The figure shows three views and two pictorial views of one solid part (mm, origin at its lowest corner). Answer the questions. A direction names the side the tool comes from. Coordinates: 2 decimals unless noted, no trailing zeros. Order: outer loops, then holes, each group sorted by start corner. A loop starts at its lowest first (then second) coordinate and runs counter-clockwise, first axis right, second up. Notation, with made-up numbers: (-10, -29.75) - (47, -29.75) arc R17 cw to (47, -15.75) - close; hole circle Ø11 at (31.25, 88.5). An arc over 180 degrees is marked (long way). Answer as a JSON object with one key per item and string values. Group by question number.
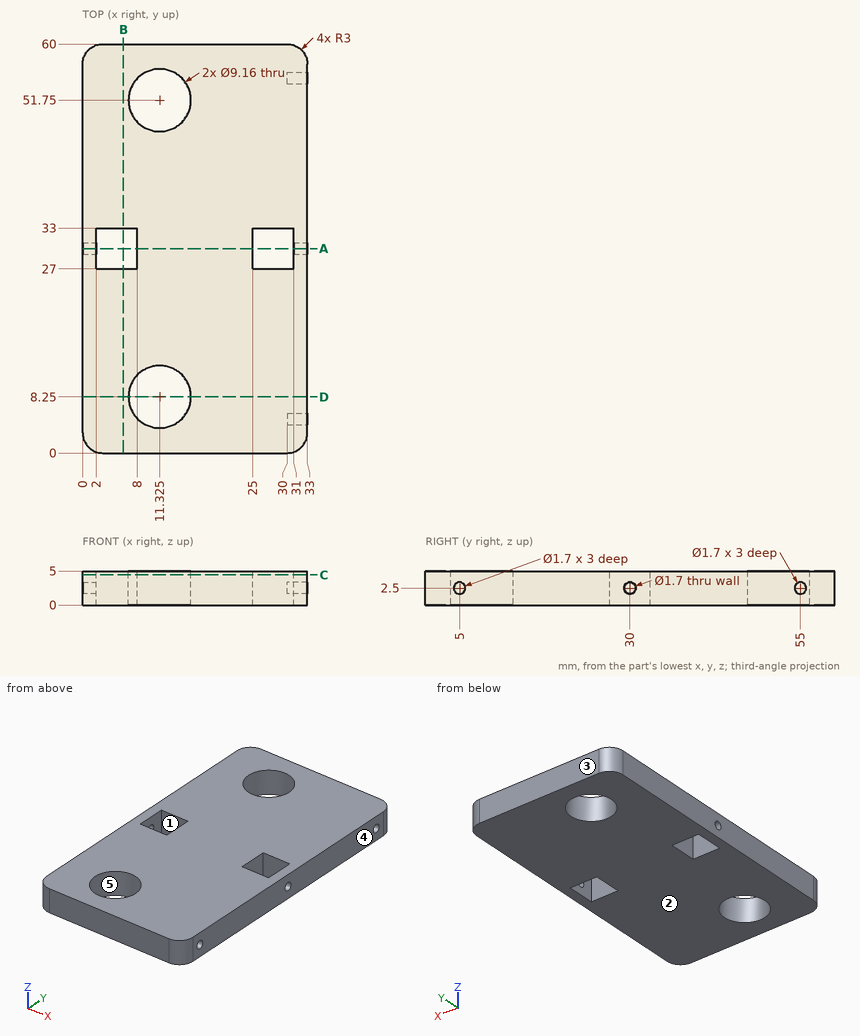
1. A cutting plane is placed at A-A on y = 30. Write down the section's boundary in (x, z).
2. For a pull along Y with two mould halves and no side action, classify the marked faces 3, 4 and 5 as pulls with the +Y half, pulls with the -Y half, needs draft (parallel to the pull), parting line crosses it, or undercut.
3. Given pin 1 (1.4 mm diameter, centred on y = 5, z = 2.5, fed in from +X); pin 2 (8 mm diameter, centred on x = 11.325, y = 51.75, fed in from +Z); pin 3 (1 mm diameter, centred on y = 30, z = 2.5, fed in from -X); pin 4 (1.4 mm diameter, centred on y = 30, z = 2.5, fed in from +X), each flat-ended and moving along its own axis, determine where each tip first touches the part or whether it passes through.
4. A cutting plane is placed at D-D on y = 8.25. Write down the section's boundary in (x, z) (3 decimals), and give its area (3 significant figures).
5. A cutting plane is placed at B-B on x = 6. Write down the section's boundary in (y, z), and give its area (3 significant figures).
6. Straight lines are drawn through the part: L1, parallel to Y at x = 11.5, z = 3.4; L2, parallel to Y at x = 26, z = 2.4; L3, parallel to X at y = 8.5, z = 1.8. For each, find the intervals that lie inside material, in ascending order.
7. For the marked faces 1 and 2, determine the directions among +Z, -Z, +X, -X, +Y, -Y from which every point of the face is accessible in a straight line to the end or side of a thin tool.
8. A cutting plane is placed at C-C on z = 4.45. Write down the section's boundary in (x, y) (3 decimals).
Derived:
{
 "1": {"outline": "(0, 0) - (2, 0) - (2, 1.65) - (0, 1.65) - close; (0, 3.35) - (2, 3.35) - (2, 5) - (0, 5) - close; (8, 0) - (25, 0) - (25, 5) - (8, 5) - close; (31, 0) - (33, 0) - (33, 1.65) - (31, 1.65) - close; (31, 3.35) - (33, 3.35) - (33, 5) - (31, 5) - close"},
 "2": {"face 3": "pulls with the +Y half", "face 4": "needs draft", "face 5": "undercut"},
 "3": {"pin 1": "stops at x = 30", "pin 2": "passes through", "pin 3": "stops at x = 8", "pin 4": "stops at x = 25"},
 "4": {"outline": "(0, 0) - (6.745, 0) - (6.745, 5) - (0, 5) - close; (15.905, 0) - (33, 0) - (33, 5) - (15.905, 5) - close", "area": "119 mm2"},
 "5": {"outline": "(0, 0) - (27, 0) - (27, 5) - (0, 5) - close; (33, 0) - (60, 0) - (60, 5) - (33, 5) - close", "area": "270 mm2"},
 "6": {"L1": "y = 0 to 3.67, 12.83 to 47.17, 56.33 to 60", "L2": "y = 0 to 27, 33 to 60", "L3": "x = 0 to 6.75, 15.9 to 33"},
 "7": {"face 1": "+Z, -Z", "face 2": "-Z, +X, -X, +Y, -Y"},
 "8": {"outline": "(0, 3) arc R3 ccw to (3, 0) - (30, 0) arc R3 ccw to (33, 3) - (33, 57) arc R3 ccw to (30, 60) - (3, 60) arc R3 ccw to (0, 57) - close; hole (2, 27) - (8, 27) - (8, 33) - (2, 33) - close; hole circle Ø9.16 at (11.325, 8.25); hole circle Ø9.16 at (11.325, 51.75); hole (25, 27) - (31, 27) - (31, 33) - (25, 33) - close"}
}
